```python
from build123d import *

# Parameters (mm, degrees)
SKIZZE1_W                       = 10.75
SKIZZE1_H                       = 5
AUFSATZ_LINEAR_AUSTRAGEN1_DEPTH = 12.75
SKIZZE2_W                       = 1.25
SKIZZE2_H                       = 1.25
AUFSATZ_LINEAR_AUSTRAGEN2_DEPTH = 8
SKIZZE3_W                       = 5.5
SKIZZE3_H                       = 0.25
AUFSATZ_LINEAR_AUSTRAGEN3_DEPTH = 2
SKIZZE4_W                       = 1.5
SKIZZE4_H                       = 1.5
SCHNITT_LINEAR_AUSTRAGEN2_DEPTH = 15.335816161
FASE1_SIZE                      = 0.25
SCHNITT_LINEAR_AUSTRAGEN3_DEPTH = 12.25
SKIZZE6_W                       = 9.5
SKIZZE6_H                       = 3.25
SCHNITT_LINEAR_AUSTRAGEN4_DEPTH = 0.125
SKIZZE7_W                       = 1.5
SKIZZE7_H                       = 3.25
SCHNITT_LINEAR_AUSTRAGEN5_DEPTH = 1
SKIZZE8_W                       = 10.75
SKIZZE8_H                       = 3.25
SCHNITT_LINEAR_AUSTRAGEN6_DEPTH = 0.125


with BuildPart() as part:
    # Skizze1 → Aufsatz-Linear austragen1 (new body)
    with BuildSketch(Plane(origin=(0, 0, 0), x_dir=(1, 0, 0), z_dir=(0, 1, 0))):
        Rectangle(SKIZZE1_W, SKIZZE1_H)
    extrude(amount=AUFSATZ_LINEAR_AUSTRAGEN1_DEPTH)

    # Skizze2 → Aufsatz-Linear austragen2 (add)
    with BuildSketch(Plane(origin=(0, 0, 0), x_dir=(1, 0, 0), z_dir=(0, 1, 0))):
        with Locations((-4.5, -3.125)):
            Rectangle(SKIZZE2_W, SKIZZE2_H)
        with Locations((2.25, -3.125)):
            Rectangle(SKIZZE2_W, SKIZZE2_H)
    extrude(amount=AUFSATZ_LINEAR_AUSTRAGEN2_DEPTH)

    # Skizze3 → Aufsatz-Linear austragen3 (add)
    with BuildSketch(Plane(origin=(0, 0, 0), x_dir=(1, 0, 0), z_dir=(0, 1, 0))):
        with Locations((-1.125, -2.625)):
            Rectangle(SKIZZE3_W, SKIZZE3_H)
    extrude(amount=AUFSATZ_LINEAR_AUSTRAGEN3_DEPTH)

    # Skizze4 → Schnitt-Linear austragen2 (cut, through all)
    with BuildSketch(Plane(origin=(0, 0, 0), x_dir=(1, 0, 0), z_dir=(0, 1, 0))):
        with Locations((-3.75, -0.875)):
            Rectangle(SKIZZE4_W, SKIZZE4_H)
        with Locations((-1.25, -0.875)):
            Rectangle(SKIZZE4_W, SKIZZE4_H)
        with Locations((1.25, -0.875)):
            Rectangle(SKIZZE4_W, SKIZZE4_H)
        with Locations((3.75, -0.875)):
            Rectangle(SKIZZE4_W, SKIZZE4_H)
    extrude(amount=SCHNITT_LINEAR_AUSTRAGEN2_DEPTH, mode=Mode.SUBTRACT)

    # Fase1
    fase1_edges = [part.edges().sort_by_distance(p)[0] for p in [
        (-4.5, 0, 0.875),
        (-3.75, 0, 1.625),
        (-3, 0, 0.875),
        (-3.75, 0, 0.125),
        (-2, 0, 0.875),
        (-1.25, 0, 1.625),
        (-0.5, 0, 0.875),
        (-1.25, 0, 0.125),
        (0.5, 0, 0.875),
        (1.25, 0, 1.625),
        (2, 0, 0.875),
        (1.25, 0, 0.125),
        (3, 0, 0.875),
        (3.75, 0, 1.625),
        (4.5, 0, 0.875),
        (3.75, 0, 0.125),
    ]]
    chamfer(fase1_edges, length=FASE1_SIZE)

    # Skizze5 → Schnitt-Linear austragen3 (cut)
    with BuildSketch(Plane(origin=(0, 12.75, 0), x_dir=(1, 0, 0), z_dir=(0, 1, 0))):
        Polygon((-4.5, 1.625), (-3, 1.625), (-3, 1.375), (-2.75, 1.375), (-2.75, -1.125), (-3, -1.125), (-3, -1.625), (-4.5, -1.625), (-4.5, -1.125), (-4.75, -1.125), (-4.75, 1.375), (-4.5, 1.375), align=None)
        Polygon((-2, 1.625), (-0.5, 1.625), (-0.5, 1.375), (-0.25, 1.375), (-0.25, -1.125), (-0.5, -1.125), (-0.5, -1.625), (-2, -1.625), (-2, -1.125), (-2.25, -1.125), (-2.25, 1.375), (-2, 1.375), align=None)
        Polygon((0.5, 1.625), (2, 1.625), (2, 1.375), (2.25, 1.375), (2.25, -1.125), (2, -1.125), (2, -1.625), (0.5, -1.625), (0.5, -1.125), (0.25, -1.125), (0.25, 1.375), (0.5, 1.375), align=None)
        Polygon((3, 1.625), (4.5, 1.625), (4.5, 1.375), (4.75, 1.375), (4.75, -1.125), (4.5, -1.125), (4.5, -1.625), (3, -1.625), (3, -1.125), (2.75, -1.125), (2.75, 1.375), (3, 1.375), align=None)
    extrude(amount=-SCHNITT_LINEAR_AUSTRAGEN3_DEPTH, mode=Mode.SUBTRACT)

    # Skizze6 → Schnitt-Linear austragen4 (cut)
    with BuildSketch(Plane(origin=(0, 12.75, 0), x_dir=(1, 0, 0), z_dir=(0, 1, 0))):
        Rectangle(SKIZZE6_W, SKIZZE6_H)
    extrude(amount=-SCHNITT_LINEAR_AUSTRAGEN4_DEPTH, mode=Mode.SUBTRACT)

    # Skizze7 → Schnitt-Linear austragen5 (cut)
    with BuildSketch(Plane(origin=(0, 0, -2.5), x_dir=(-1, 0, 0), z_dir=(0, 0, -1))):
        with Locations((-3.75, 3.125)):
            Rectangle(SKIZZE7_W, SKIZZE7_H)
        with Locations((-1.25, 3.125)):
            Rectangle(SKIZZE7_W, SKIZZE7_H)
        with Locations((1.25, 3.125)):
            Rectangle(SKIZZE7_W, SKIZZE7_H)
        with Locations((3.75, 3.125)):
            Rectangle(SKIZZE7_W, SKIZZE7_H)
    extrude(amount=-SCHNITT_LINEAR_AUSTRAGEN5_DEPTH, mode=Mode.SUBTRACT)

    # Skizze8 → Schnitt-Linear austragen6 (cut)
    with BuildSketch(Plane(origin=(0, 0, -2.5), x_dir=(-1, 0, 0), z_dir=(0, 0, -1))):
        with Locations((0, 3.125)):
            Rectangle(SKIZZE8_W, SKIZZE8_H)
    extrude(amount=-SCHNITT_LINEAR_AUSTRAGEN6_DEPTH, mode=Mode.SUBTRACT)


solid = part.part
```
Verification items for the finished model (mm, model axes). A direction names the side the tool comes from. Coordinates: 2 decimals unless noted, no trailing zeros. Loops run counter-clockwise (first coordinate to the right, second up) from the corner with the lowest first, then second, coordinate; pieces in that order, holes last. Notation, with made-up numbers: (0.5, 31) -> (58.5, 31) arc R26 ccw to (58.5, 64) -> close; hole circle Ø10 at (-19.75, -16). An arc over 180 degrees is marked (long way). Answer in a Markdown table with one row per item.
1) Section check A-A (x = 4). Record the cut outline in (y, z) (3 decimals).
The answers:
| item | result |
|---|---|
| outline | (0, -2.5) -> (1.5, -2.5) -> (1.5, -1.625) -> (0.5, -1.625) -> (0.5, 0.125) -> (0.25, 0.125) -> (0, -0.125) -> close; (0, 1.875) -> (0.25, 1.625) -> (12.75, 1.625) -> (12.75, 2.5) -> (0, 2.5) -> close; (4.75, -2.5) -> (12.75, -2.5) -> (12.75, -1.625) -> (4.75, -1.625) -> close |
2) Draft check along Y on faces 1 (the face through (-2.5, 3.1, -2.375)), 2 (the face through (-2.5, 12.625, 0)), 3 (the face through (-4.75, 7, 0)). Enter one of: released by +Y, released by -Y, zero draft, split by the parting line, or undercut.
The answers:
| item | result |
|---|---|
| face 1 | undercut |
| face 2 | released by +Y |
| face 3 | zero draft |
3) Scan lines: line 1 along X through (y, z) = (1.5, 1.5) (3 decimals); line 2 along X through (y, z) = (2.25, -0.5) (3 decimals); line 3 along Y through (x, z) = (1, -1.75). Record each from-to range of solid material in increasing order. Write a range as from..to.
The answers:
| item | result |
|---|---|
| line 1 | x = -5.375..-4.5, -3..-2, -0.5..0.5, 2..3, 4.5..5.375 |
| line 2 | x = -5.375..-4.75, -2.75..-2.25, -0.25..0.25, 2.25..2.75, 4.75..5.375 |
| line 3 | y = 0..1.5, 4.75..12.75 |
4) Access from +Z, -Z, +X, -X, +Y, -Y to the whole of each face (thin tool, end or side, straight path). Record for faces 4 (the face through (-0.5, 4, -2)), 5 (the face through (2.25, 7, 0)), 6 (the face through (-2, 6, 1.4)).
The answers:
| item | result |
|---|---|
| face 4 | none |
| face 5 | +Y |
| face 6 | +Y, -Y |
5) Section check C-C (y = 9.75). Give the number of separate pieces and of enclosed holes in the cut face, and give its area (4 significant figures).
The answers:
| item | result |
|---|---|
| separate pieces | 1 |
| enclosed holes | 4 |
| area | 29.25 mm2 |
6) Section check B-B (x = -2.5). Record the cut outline in (y, z) (3 decimals), and give its area (3 significant figures).
The answers:
| item | result |
|---|---|
| outline | (0, -2.5) -> (1.5, -2.5) -> (1.5, -2.375) -> (4.75, -2.375) -> (4.75, -2.5) -> (12.75, -2.5) -> (12.75, -1.625) -> (12.625, -1.625) -> (12.625, 1.625) -> (12.75, 1.625) -> (12.75, 2.5) -> (2, 2.5) -> (2, 2.75) -> (0, 2.75) -> close |
| area | 63.4 mm2 |
7) Depth check by flat-ended pin: P1, Ø1.4, axis at x = -4.5, z = 3, coming from the +Y side; P2, Ø1.1, axis at x = 2.5, z = 0.5, coming from the +Y side (3 decimals). Enter the tip coordinate at first touch or a pass-through.
The answers:
| item | result |
|---|---|
| P1 | stops at y = 12.75 |
| P2 | stops at y = 12.625 |
